Here's how the part is built. I have some questions about the finished solid (model axes, mm). Face numbers are marked on the shaded views. Coordinates: 2 decimals unless noted, no trailing zeros. Write each loop counter-clockwise with the first axis right and the second up, starting at its lowest first coordinate (ties: lowest second). Pieces come first, ordered by that corner, then holes. Notation, with made-up numbers: (71, 50) -> (129, 50) arc R24 ccw to (129, 78) -> close; hole circle Ø5 at (12.25, -18.5). An arc over 180 degrees is marked (long way). Put each result on its own line as item: value.
```python
from build123d import *

# Parameters (mm, degrees)
SKETCH1_W            = 112.522
SKETCH1_H            = 30.225
SKETCH2_W            = 62.484
SKETCH2_H            = 62.484
SKETCH2_R            = 3.96875
BOSS_EXTRUDE1_DEPTH  = 6.35
SKETCH3_R            = 12.7
SKETCH3_R_2          = 6.35
BOSS_EXTRUDE2_DEPTH  = 7.1374
SKETCH4_W            = 62.484
SKETCH4_H            = 62.484
BOSS_EXTRUDE3_DEPTH  = 6.35
SKETCH5_R            = 2.0828
CUT_EXTRUDE1_DEPTH   = 8.255
LPATTERN1_COUNT      = 2
LPATTERN1_PITCH      = 118.872
SKETCH6_R            = 2.0828
CUT_EXTRUDE2_DEPTH   = 6.35
LPATTERN2_COUNT      = 2
LPATTERN2_PITCH      = 43.9166
LPATTERN2_COUNT_DIR2 = 2
LPATTERN2_PITCH_DIR2 = 43.9166


with BuildPart() as part:
    # Sketch1 → Revolve1 (revolve)
    with BuildSketch(Plane(origin=(0, 0, 0), x_dir=(0, 0, -1), z_dir=(1, 0, 0)), mode=Mode.PRIVATE) as revolve1_sk:
        with Locations((56.261, -15.1125)):
            Rectangle(SKETCH1_W, SKETCH1_H)
    revolve(revolve1_sk.sketch.rotate(Axis((0, 0, 17.588251134), (0, 0, -1)), 270), axis=Axis((0, 0, 17.588251134), (0, 0, -1)))

    # Sketch2 → Boss-Extrude1 (add)
    with BuildSketch(Plane.XY):
        Rectangle(SKETCH2_W, SKETCH2_H)
        Circle(SKETCH2_R, mode=Mode.SUBTRACT)
    extrude(amount=BOSS_EXTRUDE1_DEPTH)

    # Sketch3 → Boss-Extrude2 (add)
    with BuildSketch(Plane.XY):
        with Locations(Location((0, 0, 0), (0, 0, 180))):
            Circle(SKETCH3_R)
        with Locations(Location((0, 0, 0), (0, 0, 180))):
            Circle(SKETCH3_R_2, mode=Mode.SUBTRACT)
    extrude(amount=BOSS_EXTRUDE2_DEPTH)

    # Sketch4 → Boss-Extrude3 (add)
    with BuildSketch(Plane(origin=(0, 0, -112.522), x_dir=(-1, 0, 0), z_dir=(0, 0, -1))):
        Rectangle(SKETCH4_W, SKETCH4_H)
    extrude(amount=BOSS_EXTRUDE3_DEPTH)

    # Sketch5 → Cut-Extrude1 (cut)
    with BuildSketch(Plane.XZ.offset(31.242)):
        with Locations(Location((-15.875, 3.175, 0), (0, 0, 270))):
            Circle(SKETCH5_R)
        with Locations(Location((15.875, 3.175, 0), (0, 0, 270))):
            Circle(SKETCH5_R)
    cut_extrude1 = extrude(amount=-CUT_EXTRUDE1_DEPTH, mode=Mode.SUBTRACT)

    # LPattern1: Cut-Extrude1 ×2
    with Locations(*[(0, 0, -i * LPATTERN1_PITCH) for i in range(1, LPATTERN1_COUNT)]):
        add(cut_extrude1, mode=Mode.SUBTRACT)

    # Sketch6 → Cut-Extrude2 (cut)
    with BuildSketch(Plane.XY.offset(6.35)):
        with Locations((21.9583, -21.9583)):
            Circle(SKETCH6_R)
    cut_extrude2 = extrude(amount=-CUT_EXTRUDE2_DEPTH, mode=Mode.SUBTRACT)

    # LPattern2: Cut-Extrude2 2 × 2
    with Locations(*[(-j * LPATTERN2_PITCH_DIR2, i * LPATTERN2_PITCH, 0) for i in range(LPATTERN2_COUNT) for j in range(LPATTERN2_COUNT_DIR2) if (i, j) != (0, 0)]):
        add(cut_extrude2, mode=Mode.SUBTRACT)


solid = part.part
```
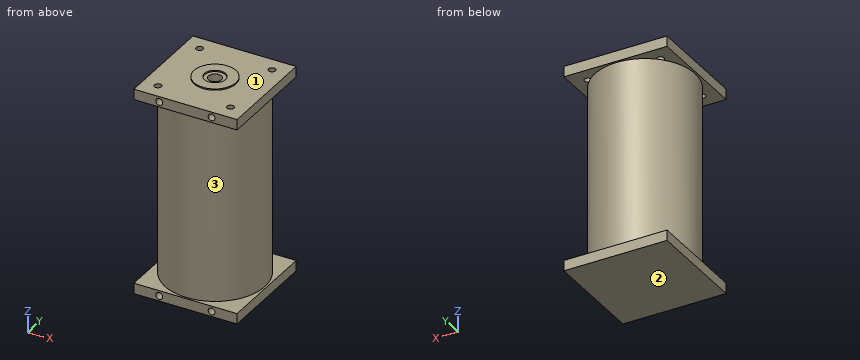
Item 1: Imagine slicing it at C-C on z = -2.5. Write out the boundary of the cut face in (x, y) (3 decimals).
Output:
outline: circle Ø60.45 at (0, 0)
Item 2: Imagine slicing it at A-A on y = 0. Write out the boundary of the cut face in (x, z) (3 decimals), then the cut area to 3 significant figures.
Output:
outline: (-31.242, -118.872) -> (31.242, -118.872) -> (31.242, -112.522) -> (30.225, -112.522) -> (30.225, 0) -> (31.242, 0) -> (31.242, 6.35) -> (12.7, 6.35) -> (12.7, 7.137) -> (6.35, 7.137) -> (6.35, 6.35) -> (3.969, 6.35) -> (3.969, 0) -> (-3.969, 0) -> (-3.969, 6.35) -> (-6.35, 6.35) -> (-6.35, 7.137) -> (-12.7, 7.137) -> (-12.7, 6.35) -> (-31.242, 6.35) -> (-31.242, 0) -> (-30.225, 0) -> (-30.225, -112.522) -> (-31.242, -112.522) -> close
area: 7,560 mm²
Item 3: Please list where these lines run through material, in increasing order: line 1 along Z through (x, y) = (27.5, 17); line 2 along Z through (x, y) = (27, 3); line 3 along X through (y, z) = (1, -95). Write a range as from..to.
Output:
line 1: z = -118.87..-112.52, 0..6.35
line 2: z = -118.87..6.35
line 3: x = -30.21..30.21
Item 4: Imagine slicing it at D-D on x = -25.5. Write out the boundary of the cut face in (y, z), then the cut area to 3 significant figures.
Output:
outline: (-31.24, -118.87) -> (31.24, -118.87) -> (31.24, -112.52) -> (16.23, -112.52) -> (16.23, 0) -> (31.24, 0) -> (31.24, 6.35) -> (-31.24, 6.35) -> (-31.24, 0) -> (-16.23, 0) -> (-16.23, -112.52) -> (-31.24, -112.52) -> close
area: 4,450 mm²
Item 5: For P1, Ø3, axis at x = -21.5, y = 21.5, coming from the +Z side; P2, Ø7.5, axis at x = 0, y = 0, coming from the +Z side; P3, Ø2, axis at x = -15.5, z = -115, coming from the -Y side; P4, Ø4.5, axis at x = 15, z = -116.5, coming from the -Y side, each with a flat end and sliding along its axis, tell me the tip position at first contact or that it passes through.
Output:
P1: stops at z = 6.35
P2: stops at z = 0
P3: stops at y = -22.99
P4: stops at y = -31.24
Item 6: If we mould it in two halves opening along Z, with no side actions, what happens to the marked faces 1, 2 and 3? For each: released by +Z, released by -Z, zero draft, split by the parting line, or undercut.
Output:
face 1: released by +Z
face 2: released by -Z
face 3: undercut
